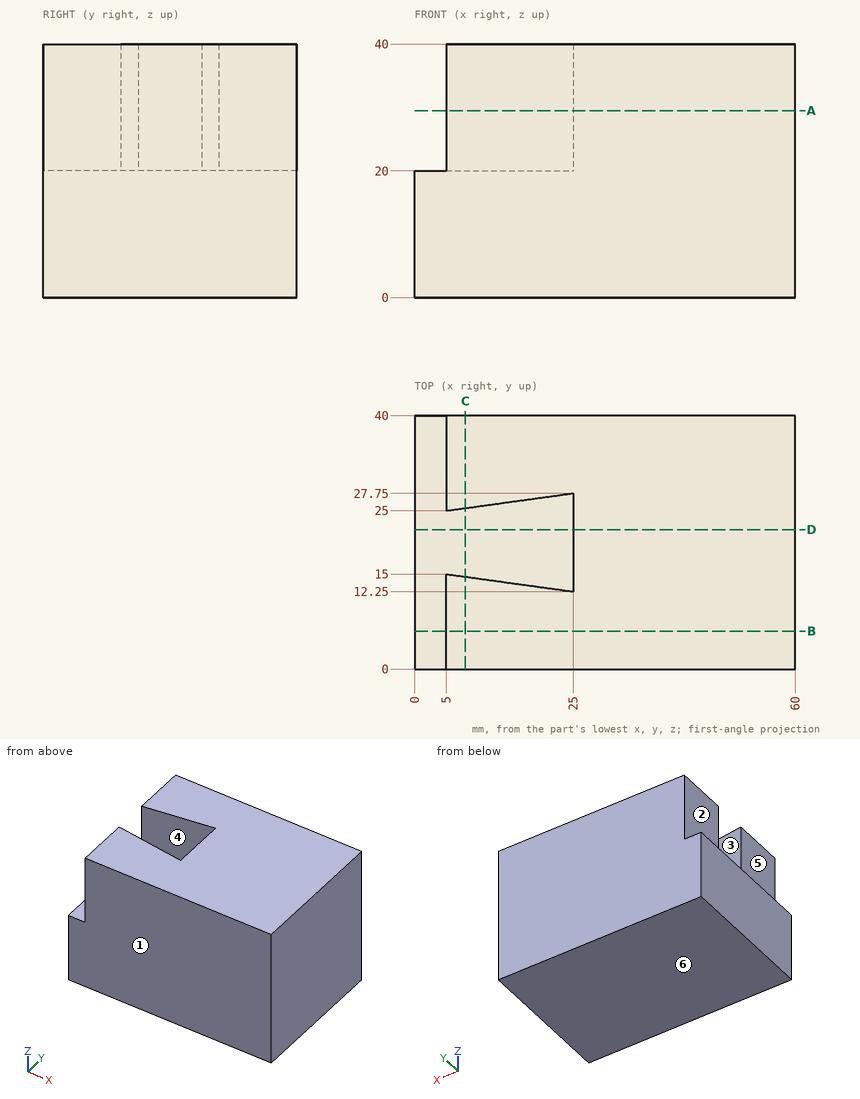
Geometry check sheet. Reference: drawing and pictorial views, mm from the part's lowest x, y, z. A direction names the side the tool comes from. Give positions to 0.01 mm unless a question says otherwise; leave off trailing zeros. Loops run counter-clockwise (first coordinate to the right, second up) from the corner with the lowest first, then second, coordinate; pieces in that order, holes last. Notation, with made-up numbers: (-11.5, -10.75) -> (26.5, -10.75) arc R11 cw to (26.5, 9.25) -> close; hole circle Ø6 at (85.5, 36.25). An arc over 180 degrees is marked (long way). Answer in a Markdown table with one row per item. Add a question column.
1) Material ranges on probe 1 along X at (y, z) = (8, 36.5); probe 2 along Z at (x, y) = (17.5, 17.5); probe 3 along Y at (x, z) = (23, 25) (3 decimals), recorded low to high. Write a range as from..to.
2) Cross-section at D-D on y = 22. Record the boundary of the cut face in (x, z).
3) Set-up check for the marked faces 4, 5 and 6: record each of +Z, -Z, +X, -X, +Y, -Y from which the full face is reachable in a straight line by a thin tool's end or side.
4) Cross-section at A-A on z = 29.5. Record the boundary of the cut face in (x, y).
5) Gauge pin test, flat end, axial feed: P1, Ø12, axis at y = 29.5, z = 29.5, coming from the -X side. Record the tip position at first contact, or that the pin passes through.
6) Cross-section at C-C on x = 8. Record the boundary of the cut face in (y, z), and give its area (3 significant figures).
7) Cross-section at B-B on y = 6. Record the boundary of the cut face in (x, z), and give its area (3 significant figures).
8) Draft check along Y on the marked faces 1, 2 and 3. Enter one of: pulls with the +Y half, pulls with the -Y half, needs draft (parallel to the pull), parting line crosses it, or undercut.
Outcome:
| question | item | result |
|---|---|---|
| 1 | probe 1 | x = 5..60 |
| 1 | probe 2 | z = 0..20 |
| 1 | probe 3 | y = 0..12.525, 27.475..40 |
| 2 | outline | (0, 0) -> (60, 0) -> (60, 40) -> (25, 40) -> (25, 20) -> (0, 20) -> close |
| 3 | face 4 | +Z |
| 3 | face 5 | +Z, -X, +Y, -Y |
| 3 | face 6 | -Z, +X, -X, +Y, -Y |
| 4 | outline | (5, 0) -> (60, 0) -> (60, 40) -> (5, 40) -> (5, 25) -> (25, 27.75) -> (25, 12.25) -> (5, 15) -> close |
| 5 | P1 | stops at x = 5 |
| 6 | outline | (0, 0) -> (40, 0) -> (40, 40) -> (25.41, 40) -> (25.41, 20) -> (14.59, 20) -> (14.59, 40) -> (0, 40) -> close |
| 6 | area | 1,380 mm^2 |
| 7 | outline | (0, 0) -> (60, 0) -> (60, 40) -> (5, 40) -> (5, 20) -> (0, 20) -> close |
| 7 | area | 2,300 mm^2 |
| 8 | face 1 | pulls with the -Y half |
| 8 | face 2 | needs draft |
| 8 | face 3 | undercut |
